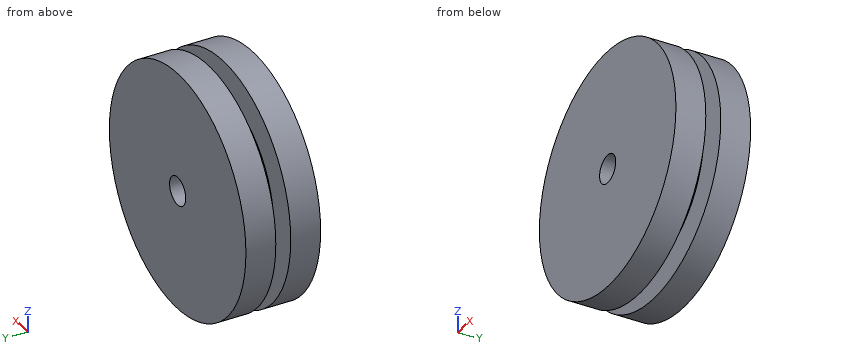
Autodesk Inventor part; units mm, degrees
ref_plane "YZ Plane" through (0, 0, 0) normal (1, 0, 0) x (0, 1, 0)
ref_plane "XZ Plane" through (0, 0, 0) normal (0, 1, 0) x (-1, 0, 0)
ref_plane "XY Plane" through (0, 0, 0) normal (0, 0, 1) x (1, 0, 0)
sketch "Sketch1" plane through (0, 0, 0) normal (0, 1, 0) x (-1, 0, 0)
  circle A0 centre (0, 0) radius 25.4
  dimension "d0" = 50.8
extrude "Extrusion1" add sketch "Sketch1" along normal blind 6.35
sketch "Sketch2" plane through (0, 6.35, 0) normal (0, 1, 0) x (1, 0, 0)
  circle A0 centre (0, 0) radius 19.05
  dimension "d3" = 38.1
extrude "Extrusion2" add sketch "Sketch2" along normal blind 3.175
sketch "Sketch3" plane through (0, 9.525, 0) normal (0, 1, 0) x (1, 0, 0)
  circle A0 centre (0, 0) radius 25.4
extrude "Extrusion3" add sketch "Sketch3" along normal blind 6.35
sketch "Sketch5" plane through (0, 15.875, 0) normal (0, 1, 0) x (1, 0, 0)
  circle A0 centre (0, 0) radius 3
  dimension "d10" = 6
hole "Hole1" at (0, 15.875, 0) direction (0, -1, 0) diameter 6 end through all
properties part number "Wheel_design"
Verification items for the finished model (mm, model axes). Coordinates: 2 decimals unless noted, no trailing zeros. Loops run counter-clockwise (first coordinate to the right, second up) from the corner with the lowest first, then second, coordinate; pieces in that order, holes last. Notation, with made-up numbers: (-11.75, 55.25) - (31.25, 55.25) arc R17 cw to (31.25, 80.25) - close; hole circle Ø6 at (89, 37.25). An arc over 180 degrees is marked (long way). Put each result on its own line as item: value.
Item 1: Section check A-A (z = 0). Enter the section's corners in (x, y) (3 decimals).
Conclusion:
outline: (-25.4, 0) - (-3, 0) - (-3, 15.875) - (-25.4, 15.875) - (-25.4, 9.525) - (-19.05, 9.525) - (-19.05, 6.35) - (-25.4, 6.35) - close; (3, 0) - (25.4, 0) - (25.4, 6.35) - (19.05, 6.35) - (19.05, 9.525) - (25.4, 9.525) - (25.4, 15.875) - (3, 15.875) - close
Item 2: Section check B-B (x = 0). Enter the section's corners in (y, z) (3 decimals), then the cut area to 3 significant figures.
Conclusion:
outline: (0, -25.4) - (6.35, -25.4) - (6.35, -19.05) - (9.525, -19.05) - (9.525, -25.4) - (15.875, -25.4) - (15.875, -3) - (0, -3) - close; (0, 3) - (15.875, 3) - (15.875, 25.4) - (9.525, 25.4) - (9.525, 19.05) - (6.35, 19.05) - (6.35, 25.4) - (0, 25.4) - close
area: 671 mm2
Item 3: Section check D-D (x = 16). Enter the section's corners in (y, z) (3 decimals).
Conclusion:
outline: (0, -19.727) - (6.35, -19.727) - (6.35, -10.339) - (9.525, -10.339) - (9.525, -19.727) - (15.875, -19.727) - (15.875, 19.727) - (9.525, 19.727) - (9.525, 10.339) - (6.35, 10.339) - (6.35, 19.727) - (0, 19.727) - close
Item 4: Scan lines: line 1 along Z through (x, y) = (0, 8); line 2 along Z through (x, y) = (0, 10.25). Record each from-to range of solid material in increasing order.
Conclusion:
line 1: z = -19.05 to -3, 3 to 19.05
line 2: z = -25.4 to -3, 3 to 25.4
Item 5: Section check C-C (y = 3.25). Enter the section's corners in (x, z), then the cut area to 3 significant figures.
Conclusion:
outline: circle Ø50.8 at (0, 0); hole circle Ø6 at (0, 0)
area: 2,000 mm2
Item 6: Gauge pin test, flat ends, axial feed: pin 1 Ø1.5 at (y, z) = (5, 10.5) entering from -X; pin 2 Ø1 at (x, y) = (-15.5, 5.5) entering from -Z; pin 3 Ø5 at (x, y) = (-3, 13.5) entering from +Z. Record the tip position at first contact, or that the pin passes through.
Conclusion:
pin 1: stops at x = -23.45
pin 2: stops at z = -20.5
pin 3: stops at z = 25.4
